The listing builds one solid part. Answer for the finished solid, in the listing's coordinates (mm). A direction names the side the tool comes from. Coordinates: 2 decimals unless noted, no trailing zeros. Write each loop counter-clockwise with the first axis right and the second up, starting at its lowest first coordinate (ties: lowest second). Pieces come first, ordered by that corner, then holes.
Autodesk Inventor part; units mm, degrees
sketch "Sketch1" plane through (0, 0, 0) normal (0, 0, 1) x (1, 0, 0)
  line L0 (0, 2.8582) -> (0, -2.8582) construction
  line L1 (-5.7775, 0) -> (5.7775, 0) construction
  circle A0 centre (0, 0) radius 25.629
  circle A1 centre (0, 0) radius 4
  line L2 (0, 4) -> (0, 7)
  line L3 (0, 7) -> (0, 21)
  line L4 (0, 21) -> (5, 21)
  line L5 (5, 21) -> (8, 21)
  line L6 (8, 21) -> (0, 7)
  line L7 (0, 21) -> (-8, 21)
  line L8 (-8, 21) -> (0, 7)
  line L9 (0, -4) -> (0, -7)
  line L10 (0, -7) -> (0, -21)
  line L11 (0, -21) -> (8, -21)
  line L12 (8, -21) -> (0, -7)
  line L13 (0, -21) -> (-8, -21)
  line L14 (-8, -21) -> (0, -7)
  line L15 (0, 0) -> (2.5981, 1.5)
  line L16 (0, 0) -> (3, 0) construction
  line L17 (2.5981, 1.5) -> (3.4641, 2)
  line L18 (3.4641, 2) -> (6.0622, 3.5)
  line L19 (6.0622, 3.5) -> (18.1865, 10.5)
  line L20 (18.1865, 10.5) -> (14.1865, 17.4282)
  line L21 (14.1865, 17.4282) -> (6.0622, 3.5)
  line L22 (18.1865, 10.5) -> (22.1865, 3.5718)
  line L23 (22.1865, 3.5718) -> (6.0622, 3.5)
  line L24 (0, 0) -> (8, 0) construction
  line L25 (0, 0) -> (3.4641, -2)
  line L26 (0, 0) -> (4, 0) construction
  line L27 (3.4641, -2) -> (6.0622, -3.5)
  line L28 (6.0622, -3.5) -> (18.1865, -10.5)
  line L29 (18.1865, -10.5) -> (14.1865, -17.4282)
  line L30 (14.1865, -17.4282) -> (6.0934, -3.518)
  line L31 (18.1865, -10.5) -> (22.0919, -3.518)
  line L32 (22.0919, -3.518) -> (6.0934, -3.518)
  line L33 (0, 0) -> (-2.5981, 1.5)
  line L34 (0, 0) -> (3, 0) construction
  line L35 (-2.5981, 1.5) -> (-3.4641, 2)
  line L36 (-3.4641, 2) -> (-6.0622, 3.5)
  line L37 (-6.0622, 3.5) -> (-18.1865, 10.5)
  line L38 (-18.1865, 10.5) -> (-14.1865, 17.4282)
  line L39 (-14.1865, 17.4282) -> (-6.0622, 3.5)
  line L40 (-18.1865, 10.5) -> (-22.1865, 3.5718)
  line L41 (-22.1865, 3.5718) -> (-6.0622, 3.5)
  line L42 (0, 0) -> (-6.0622, -3.5)
  line L43 (0, 0) -> (7, 0) construction
  line L44 (-6.0622, -3.5) -> (-18.1865, -10.5)
  line L45 (-18.1865, -10.5) -> (-14.1865, -17.4282)
  line L46 (-14.1865, -17.4282) -> (-6.0622, -3.5)
  line L47 (-18.1865, -10.5) -> (-22.1865, -3.5718)
  line L48 (-22.1865, -3.5718) -> (-6.0622, -3.5)
  dimension "d0" = 51.258
  dimension "d1" = 8
  dimension "d2" = 3
  dimension "d3" = 14
  dimension "d4" = 5
  dimension "d5" = 3
  dimension "d6" = 8
  dimension "d7" = 3
  dimension "d8" = 14
  dimension "d9" = 8
  dimension "d10" = 8
  dimension "d11" = 3
  dimension "d12" = 30
  dimension "d13" = 3
  dimension "d14" = 14
  dimension "d15" = 8
  dimension "d16" = 8
  dimension "d19" = 4
  dimension "d20" = 30
  dimension "d21" = 3
  dimension "d22" = 14
  dimension "d23" = 8
  dimension "d24" = 8
  dimension "d25" = 3
  dimension "d26" = 150
  dimension "d27" = 1
  dimension "d28" = 180
  dimension "d29" = 3
  dimension "d30" = 180
  dimension "d31" = 180
  dimension "d32" = 8
  dimension "d33" = 8
  dimension "d34" = 7
  dimension "d35" = 150
  dimension "d36" = 14
  dimension "d37" = 180
  dimension "d38" = 8
  dimension "d39" = 8
extrude "Extrusion1" add sketch "Sketch1" along normal blind 2
fillet "Fillet1" radius 2 18 edges at (14.1865, 17.4282, 1) (22.1865, 3.5718, 1) (6.0622, 3.5, 1) (22.0919, -3.518, 1) (14.1865, -17.4282, 1) (6.0934, -3.518, 1) (0, 7, 1) (-8, 21, 1) (8, 21, 1) (-6.0622, 3.5, 1) (-22.1865, 3.5718, 1) (-14.1865, 17.4282, 1) (-6.0622, -3.5, 1) (-14.1865, -17.4282, 1) (-22.1865, -3.5718, 1) (-8, -21, 1) (0, -7, 1) (8, -21, 1)
sketch "Sketch2" plane through (0, 0, 2) normal (0, 0, 1) x (1, 0, 0)
  circle A0 centre (0, 0) radius 3.05
  circle A1 centre (0, 0) radius 5
  dimension "d43" = 6.1
  dimension "d49" = 10
extrude "Extrusion2" add sketch "Sketch2" against normal blind 2
chamfer "Chamfer1" distance 1 angle 45 1 edges at (-25.629, 0, 2)
sketch "Sketch4" plane through (0, 0, 2) normal (0, 0, 1) x (1, 0, 0)
  circle A0 centre (0, 0) radius 3.05
  circle A1 centre (0, 0) radius 6
  dimension "d54" = 6.1
  dimension "d55" = 12
extrude "Extrusion4" add sketch "Sketch4" along normal blind 20
fillet "Fillet2" radius 2 1 edges at (-6, 0, 2)
properties part number "Wiel hout+spacer" material "S235"
1. Section C-C on z = 15.25 is taken. Give the vertices of the cut face in (x, y), then the cut area to 3 significant figures.
Results found:
outline: circle Ø12 at (0, 0); hole circle Ø6.1 at (0, 0)
area: 83.9 mm2
2. Flat-ended cylindrical pins translate along their axes: P1, Ø10, axis at x = -10.5, z = 2.5, coming from the -Y side; P2, Ø12, axis at y = -6, z = 7.5, coming from the -X side; P3, Ø0.6, axis at x = 0, z = 1.5, coming from the -Y side; P4, Ø2, axis at x = 0.5, y = 10.5, coming from the -Z side. Find the tip coordinate at first contact, or state that the pin passes through.
Results found:
P1: stops at y = -24.98
P2: stops at x = -24.54
P3: stops at y = -25.43
P4: passes through
3. Find the intervals of material crossed by L1, parallel to Y at x = 0, z = 11; L2, parallel to Z at x = -19, y = 10; L3, parallel to X at y = 16, z = 1, in increasing order.
Results found:
L1: y = -6 to -3.05, 3.05 to 6
L2: z = 0 to 2
L3: x = -20.02 to -5.14, 5.14 to 20.02
4. Section A-A on x = 0 is taken. Give the vertices of the cut face in (y, z), then the cut area to 3 significant figures.
Results found:
outline: (-25.63, 0) - (-21, 0) - (-21, 2) - (-24.63, 2) - (-25.63, 1) - close; (-9.03, 0) - (-3.05, 0) - (-3.05, 22) - (-6, 22) - (-6, 4) arc R2 cw to (-8, 2) - (-9.03, 2) - close; (3.05, 0) - (9.03, 0) - (9.03, 2) - (8, 2) arc R2 cw to (6, 4) - (6, 22) - (3.05, 22) - close; (21, 0) - (25.63, 0) - (25.63, 1) - (24.63, 2) - (21, 2) - close
area: 161 mm2
5. Section D-D on x = 19.5 is taken. State how many separate pieces and enclosed holes the cut face has, then the cut area to 3 significant figures.
Results found:
separate pieces: 3
enclosed holes: 0
area: 47.0 mm2
6. Section B-B on y = 0 is taken. Give the vertices of the cut face in (x, z).
Results found:
outline: (-25.63, 0) - (-3.05, 0) - (-3.05, 22) - (-6, 22) - (-6, 4) arc R2 cw to (-8, 2) - (-24.63, 2) - (-25.63, 1) - close; (3.05, 0) - (25.63, 0) - (25.63, 1) - (24.63, 2) - (8, 2) arc R2 cw to (6, 4) - (6, 22) - (3.05, 22) - close
7. For a pull along Y with two mould halves and no side action, classify faces 1 (the cylindrical face through (-6, 0, 13)), 2 (the flat face through (0, -21, 1)), 3 (the cylindrical face through (-14.211, -15.443, 1.014)), 4 (the flat face through (3, -3, 22)) as pulls with the +Y half, pulls with the -Y half, needs draft (parallel to the pull), parting line crosses it, or undercut.
Results found:
face 1: parting line crosses it
face 2: undercut
face 3: undercut
face 4: needs draft
8. A tool of negligible diameter and unlimited length cuts with its end or side. For faces 5 (the flat face through (-4, -14, 1)), 6 (the flat face through (-6, 6, 2)), from which of +Z, -Z, +X, -X, +Y, -Y can it reach the whole face along a straight path? Write none if from no direction.
Results found:
face 5: +Z, -Z
face 6: +Z
